CAD build for the part. Positions are in the model's coordinates, mm. A direction names the side the tool comes from. Coordinates: 2 decimals unless noted, no trailing zeros. Write each loop counter-clockwise with the first axis right and the second up, starting at its lowest first coordinate (ties: lowest second). Pieces come first, ordered by that corner, then holes.
Autodesk Inventor part; units mm, degrees
ref_plane "YZ Plane" through (0, 0, 0) normal (1, 0, 0) x (0, 1, 0)
sketch "Sketch1" plane through (0, 0, 0) normal (0, 0, 1) x (1, 0, 0)
  line L0 (6.5, -9.3) -> (385, -9.3)
  line L1 (400, -24.3) -> (400, -135)
  line L2 (385, -150) -> (-400, -150)
  line L3 (-400, -150) -> (-400, -32.4)
  line L4 (6.5, -9.3) -> (6.5, -13.8)
  line L5 (6.5, -13.8) -> (380.5, -13.8)
  line L6 (395.5, -28.8) -> (395.5, -130.5)
  line L7 (380.5, -145.5) -> (-395.5, -145.5)
  line L8 (-400, -32.4) -> (375.5, -32.4)
  line L9 (390.5, -47.4) -> (390.5, -122.25)
  line L10 (375.5, -137.25) -> (-387.25, -137.25)
  line L11 (-395.5, -145.5) -> (-395.5, -36.9)
  line L12 (-395.5, -36.9) -> (371, -36.9)
  line L13 (386, -51.9) -> (386, -117.75)
  line L14 (371, -132.75) -> (-382.75, -132.75)
  line L15 (-382.75, -132.75) -> (-382.75, -60)
  line L16 (-387.25, -137.25) -> (-387.25, -55.5)
  line L17 (-387.25, -55.5) -> (366, -55.5)
  line L18 (381, -70.5) -> (381, -109.5)
  line L19 (-382.75, -60) -> (361.5, -60)
  line L20 (376.5, -75) -> (376.5, -105)
  line L21 (361.5, -120) -> (-374.5, -120)
  line L22 (366, -124.5) -> (-374.5, -124.5)
  line L23 (-374.5, -124.5) -> (-374.5, -120)
  arc A0 (400, -24.3) -> (385, -9.3) centre (385, -24.3) ccw
  arc A1 (395.5, -28.8) -> (380.5, -13.8) centre (380.5, -28.8) ccw
  arc A2 (390.5, -47.4) -> (375.5, -32.4) centre (375.5, -47.4) ccw
  arc A3 (386, -51.9) -> (371, -36.9) centre (371, -51.9) ccw
  arc A4 (381, -70.5) -> (366, -55.5) centre (366, -70.5) ccw
  arc A5 (376.5, -75) -> (361.5, -60) centre (361.5, -75) ccw
  arc A6 (361.5, -120) -> (376.5, -105) centre (361.5, -105) ccw
  arc A7 (366, -124.5) -> (381, -109.5) centre (366, -109.5) ccw
  arc A8 (371, -132.75) -> (386, -117.75) centre (371, -117.75) ccw
  arc A9 (375.5, -137.25) -> (390.5, -122.25) centre (375.5, -122.25) ccw
  arc A10 (380.5, -145.5) -> (395.5, -130.5) centre (380.5, -130.5) ccw
  arc A11 (385, -150) -> (400, -135) centre (385, -135) ccw
  line L24 (322.4983, 0) -> (322.4983, -162)
  line L25 (322.4983, -162) -> (407.2483, -162)
  line L26 (407.2483, -162) -> (407.2483, 0)
  line L27 (407.2483, 0) -> (322.4983, 0)
  line L28 (-561.4497, 0) -> (568.6979, 0)
  line L29 (322.4983, -123.614) -> (322.4983, -76.5697)
  line L30 (322.4983, -65.8872) -> (366.8197, -65.8872)
  line L31 (366.8197, -65.8872) -> (366.8197, -114.4349)
  line L32 (366.8197, -114.4349) -> (322.4983, -114.4349)
  point P0 (0, 0)
  point P1 (400, -9.3)
  point P2 (400, -150)
  point P3 (395.5, -13.8)
  point P4 (395.5, -145.5)
  point P5 (390.5, -32.4)
  point P6 (390.5, -137.25)
  point P7 (386, -36.9)
  point P8 (386, -132.75)
  point P9 (381, -55.5)
  point P10 (381, -124.5)
  point P11 (376.5, -60)
  point P12 (376.5, -120)
  point P13 (0, 0)
  point P14 (322.4983, -60)
  point P15 (322.4983, -120)
  point P16 (322.4983, -36.9)
  point P17 (322.4983, -55.5)
  point P18 (322.4983, -124.5)
  point P19 (322.4983, -132.75)
  point P20 (322.4983, -13.8)
  point P21 (322.4983, -32.4)
  point P22 (322.4983, -137.25)
  point P23 (322.4983, -145.5)
  point P24 (322.4983, -150)
  point P25 (322.4983, -9.3)
  dimension "d1" = 4.5
  dimension "d2" = 4.5
  dimension "d3" = 4.5
  dimension "d5" = 800
  dimension "d6" = 400
  dimension "d7" = 4.5
  dimension "d8" = 4.5
  dimension "d9" = 5
  dimension "d10" = 4.5
  dimension "d11" = 18.6
  dimension "d12" = 4.5
  dimension "d13" = 8.25
  dimension "d14" = 4.5
  dimension "d15" = 4.5
  dimension "d16" = 4.5
  dimension "d17" = 5
  dimension "d19" = 18.6
  dimension "d20" = 8.25
  dimension "d89" = 8.25
  dimension "d90" = 8.25
  dimension "d91" = 15
  dimension "d104" = 84.75
  dimension "d106" = 162
extrude "Extrusion1" add sketch "Sketch1" along normal blind 4.5 contours L24 L27 L26 L25 L2 A11 L1 A0 L0 | L5 A1 L6 A10 L7 L24 L10 A9 L9 A2 L8 | L12 A3 L13 A8 L14 L24 L22 A7 L18 A4 L17 | L19 A5 L20 A6 L21 L24 L32 L31 L30
extrude "Extrusion7" add sketch "Sketch1" against normal blind 0.45 contours L24 L27 L26 L25 L2 A11 L1 A0 L0 | L0 A0 L1 A11 L2 L24 L7 A10 L6 A1 L5 | L5 A1 L6 A10 L7 L24 L10 A9 L9 A2 L8 | L8 A2 L9 A9 L10 L24 L14 A8 L13 A3 L12 | L12 A3 L13 A8 L14 L24 L22 A7 L18 A4 L17 | L17 A4 L18 A7 L22 L24 L21 A6 L20 A5 L19 | L19 A5 L20 A6 L21 L24 L32 L31 L30 | L30 L31 L32 L24
equation "\"d1\" = wire_diameter"
equation "\"d2\" = wire_diameter"
equation "\"d3\" = wire_diameter"
equation "\"d5\" = track_length"
equation "\"d7\" = wire_diameter"
equation "\"d8\" = wire_diameter"
equation "\"d10\" = wire_diameter"
equation "\"d11\" = distance_between_wires"
equation "\"d12\" = wire_diameter"
equation "\"d13\" = distance_between_wires_edge"
equation "\"d14\" = wire_diameter"
equation "\"d15\" = wire_diameter"
equation "\"d16\" = wire_diameter"
equation "\"d19\" = distance_between_wires"
equation "\"d20\" = distance_between_wires_edge"
equation "\"d22\" = wire_diameter"
equation "\"track_length\" = 800"
equation "\"wire_diameter\" = 4.5"
equation "\"distance_between_wires\" = -1.2 * wire_diameter + 0.2 * parameter_6"
equation "\"distance_between_wires_edge\" = 8.25"
equation "\"bend_radius\" = 15"
properties part number "primary_coil_0R2_test_cut"
Item 1: Saw through at D-D, the plane y = -43.5. Write the cut outline in (x, z).
Item 2: Flat gauge pins, fed straight in: pin 1 Ø2 at (x, z) = (348, 3) entering from +Y; pin 2 Ø2 at (y, z) = (-99.5, 2) entering from -X; pin 3 Ø4 at (x, y) = (355.5, -90.5) entering from +Z. Where does each tip first touch, or does it go through?
Item 3: Wall check: line 1 along X through (y, z) = (-89, 0.9); line 2 along X through (y, z) = (-120.5, 3.5); line 3 along X through (y, z) = (-108.5, 1.2). Give the ranges that are in metal, low to high.
Item 4: Saw through at A-A, the plane y = -86. Write the cut outline in (x, z).
Item 5: Two-plate mould, pull along Y, no slides. Class faces 1 (the flat face through (382, -74, 4.5)), 2 (the flat face through (364, -162, 2)), 3 (the cylindrical face through (390.99, -18.08, 2.22)), 4 (the cylindrical face through (376.49, -59.78, 2.22)): +Y half, -Y half, draft (parallel to the pull), parting line (faces both ways), or undercut.
Item 6: Saw through at B-B, the plane z = 2.75. State how many separate pieces and enclosed holes the cut face has, and give its area (3 significant figures).
Item 7: Saw through at C-C, the plane x = 387.5. Write the cut outline in (y, z).
Item 8: Which spindle directions (+Z, -Z, +X, -X, +Y, -Y) get a long thin tool onto all of the face, cutting with end or side? Do faces 5 (the flat face through (354, -150, 2)), 6 (the flat face through (390.5, -84, 2)), 7 (the flat face through (402, -87, 4.5)). Say none if no direction does.
Working result:
1. outline: (322.5, -0.45) - (407.25, -0.45) - (407.25, 4.5) - (400, 4.5) - (400, 0) - (395.5, 0) - (395.5, 4.5) - (389.98, 4.5) - (389.98, 0) - (383.43, 0) - (383.43, 4.5) - (322.5, 4.5) - close
2. pin 1: stops at y = 0
2. pin 2: stops at x = 366.82
2. pin 3: stops at z = 0
3. line 1: x = 366.82 to 376.5, 381 to 386, 390.5 to 395.5, 400 to 407.25
3. line 2: x = 376.2 to 385.75, 390.5 to 395.5, 400 to 407.25
3. line 3: x = 366.82 to 376.09, 381 to 386, 390.5 to 395.5, 400 to 407.25
4. outline: (322.5, -0.45) - (407.25, -0.45) - (407.25, 4.5) - (400, 4.5) - (400, 0) - (395.5, 0) - (395.5, 4.5) - (390.5, 4.5) - (390.5, 0) - (386, 0) - (386, 4.5) - (381, 4.5) - (381, 0) - (376.5, 0) - (376.5, 4.5) - (366.82, 4.5) - (366.82, 0) - (322.5, 0) - close
5. face 1: draft
5. face 2: -Y half
5. face 3: undercut
5. face 4: undercut
6. separate pieces: 4
6. enclosed holes: 0
6. area: 8,450 mm2
7. outline: (-162, -0.45) - (0, -0.45) - (0, 4.5) - (-9.51, 4.5) - (-9.51, 0) - (-15.53, 0) - (-15.53, 4.5) - (-38.4, 4.5) - (-38.4, 0) - (-131.25, 0) - (-131.25, 4.5) - (-143.77, 4.5) - (-143.77, 0) - (-149.79, 0) - (-149.79, 4.5) - (-162, 4.5) - close
8. face 5: +Z, -X
8. face 6: +Z
8. face 7: +Z, +X, -X, +Y, -Y
